Read the model definition and answer for the solid it produces. Units are mm, in the model's axes. A direction names the side the tool comes from. Coordinates: 2 decimals unless noted, no trailing zeros. Loops run counter-clockwise (first coordinate to the right, second up) from the corner with the lowest first, then second, coordinate; pieces in that order, holes last. Notation, with made-up numbers: (62, 62.5) - (120, 62.5) arc R13 cw to (120, 73.5) - close; hole circle Ø7 at (69.5, 77.5). An arc over 180 degrees is marked (long way). Use one line per item in the form item = value. Start each with the question number.
1) Each of these flat-tipped pins is pushed along its axis until it touches: P1, Ø1.5, axis at y = 1, z = 0, coming from the +X side; P2, Ø1.2, axis at x = 8.5, y = 2, coming from the -Z side. Where does it stop, or does it pass through?
2) The mould has two halves that part along X. Classify faces 1 (the face through (-2.017, 2.028, 9.283)), 2 (the face through (-0.397, 1.972, -17.024)), 3 (the face through (5.046, 1.972, -12.871)): released by +X, released by -X, zero draft, split by the parting line, or undercut.
3) Which of the six approach directions +Z, -Z, +X, -X, +Y, -Y give full straight-line access (tool end or side, diameter ignored) to faces 4 (the face through (9.56, 2.03, -6.91)), 5 (the face through (-5.11, 2.03, -0.39)), 6 (the face through (8, 2, -10.309))?
4) A cutting plane is placed at D-D (z = 5.75). Give the vertices of the cut face in (x, y), and give its area (3 significant figures).
5) A cutting plane is placed at C-C (x = -5.75). Give the vertices of the cut face in (y, z), and give its area (3 significant figures).
6) A cutting plane is placed at A-A (z = 0). Give the vertices of the cut face in (x, y).
7) A cutting plane is placed at B-B (y = 2.45). Give the vertices of the cut face in (x, z), and give its area (3 significant figures).
8) Consider line 1 (X direction, y = 0.9, z = 0); line 2 (Z direction, x = 0, y = 2.85); line 3 (Z direction, x = 0.5, y = 0.2). Determine where each line is inside the solid, lowest interval first.
from build123d import *

# Parameters (mm, degrees)
SKETCH1_R           = 3.05
SKETCH1_R_2         = 2.5
BOSS_EXTRUDE1_DEPTH = 4
SKETCH2_R           = 1.3
CUT_EXTRUDE1_DEPTH  = 4
SKETCH3_R           = 7.65
BOSS_EXTRUDE2_DEPTH = 4
BOSS_EXTRUDE3_DEPTH = 4
FILLET9_R           = 0.5


with BuildPart() as part:
    # Sketch1 → Boss-Extrude1 (new body)
    with BuildSketch(Plane(origin=(0, 0, 0), x_dir=(1, 0, 0), z_dir=(0, 1, 0))):
        with BuildLine():
            Line((-4.488689239, 15.114947499), (-7.764071496, 1.928521143))
            ThreePointArc((-7.764071496, 1.928521143), (0, -8), (7.764071496, 1.928521143))
            Line((7.764071496, 1.928521143), (4.488689239, 15.114947499))
            ThreePointArc((4.488689239, 15.114947499), (0, 18.625088), (-4.488689239, 15.114947499))
        make_face()
        with Locations((0, 14)):
            Circle(SKETCH1_R, mode=Mode.SUBTRACT)
        Circle(SKETCH1_R_2, mode=Mode.SUBTRACT)
    extrude(amount=BOSS_EXTRUDE1_DEPTH)

    # Sketch2 → Cut-Extrude1 (cut)
    with BuildSketch(Plane(origin=(0, 4, 0), x_dir=(1, 0, 0), z_dir=(0, 1, 0))):
        with Locations((0, 6.35)):
            Circle(SKETCH2_R)
        with Locations((6.35, 0)):
            Circle(SKETCH2_R)
        with Locations((0, -6.35)):
            Circle(SKETCH2_R)
        with Locations((-6.35, 0)):
            Circle(SKETCH2_R)
    extrude(amount=-CUT_EXTRUDE1_DEPTH, mode=Mode.SUBTRACT)

    # Sketch3 → Boss-Extrude2 (add)
    with BuildSketch(Plane(origin=(0, 4, 0), x_dir=(1, 0, 0), z_dir=(0, 1, 0))):
        with BuildLine():
            ThreePointArc((-1.549317863, 9.3728125), (0, -9.5), (1.549317863, 9.3728125))
            ThreePointArc((1.549317863, 9.3728125), (0, 9.120322757), (-1.549317863, 9.3728125))
        make_face()
        Circle(SKETCH3_R, mode=Mode.SUBTRACT)
    extrude(amount=-BOSS_EXTRUDE2_DEPTH)

    # Sketch4 → Boss-Extrude3 (add)
    with BuildSketch(Plane(origin=(0, 4, 0), x_dir=(1, 0, 0), z_dir=(0, 1, 0))):
        with BuildLine():
            Line((10.767160229, 10.309478294), (8.567165836, 4.1053221))
            Line((8.567165836, 4.1053221), (2.165063509, 1.25))
            ThreePointArc((2.165063509, 1.25), (1.994303817, 1.507565019), (1.793071605, 1.742094779))
            Line((1.793071605, 1.742094779), (5.682321854, 10.309478294))
            Line((5.682321854, 10.309478294), (10.767160229, 10.309478294))
        make_face()
    extrude(amount=-BOSS_EXTRUDE3_DEPTH)

    # Fillet9
    fillet9_edges = [part.edges().sort_by_distance(p)[0] for p in [
        (5.682321854, 2, -10.309478294),
        (10.767160229, 2, -10.309478294),
    ]]
    fillet(fillet9_edges, radius=FILLET9_R)


solid = part.part
Found:
q1.P1 = 9.5
q1.P2 = -10.31
q2.face_1 = split by the parting line
q2.face_2 = undercut
q2.face_3 = released by +X
q3.face_4 = +X, +Y, -Y
q3.face_5 = +Y, -Y
q3.face_6 = -Z, +X, +Y, -Y
q4.outline = (-7.56, 0) - (-1.15, 0) - (-1.15, 4) - (-7.56, 4) - close; (1.15, 0) - (7.56, 0) - (7.56, 4) - (1.15, 4) - close
q4.area = 51.3 mm^2
q5.outline = (0, -10.04) - (4, -10.04) - (4, -1.15) - (0, -1.15) - close; (0, 1.15) - (4, 1.15) - (4, 7.56) - (0, 7.56) - close
q5.area = 61.2 mm^2
q6.outline = (-9.5, 0) - (-7.65, 0) - (-7.65, 4) - (-9.5, 4) - close; (-5.05, 0) - (-2.5, 0) - (-2.5, 4) - (-5.05, 4) - close; (2.5, 0) - (5.05, 0) - (5.05, 4) - (2.5, 4) - close; (7.65, 0) - (9.5, 0) - (9.5, 4) - (7.65, 4) - close
q7.outline = (-6.53, -6.9) - (-4.49, -15.11) arc R4.63 ccw to (4.49, -15.11) - (5.59, -10.69) arc R0.5 cw to (6.07, -10.31) - (10.06, -10.31) arc R0.5 ccw to (10.53, -9.64) - (8.57, -4.11) arc R9.5 ccw (long way) to start; hole circle Ø2.6 at (-6.35, 0); hole circle Ø6.1 at (0, -14); hole circle Ø5 at (0, 0); hole circle Ø2.6 at (0, -6.35); hole circle Ø2.6 at (0, 6.35); hole circle Ø2.6 at (6.35, 0)
q7.area = 322 mm^2
q8.line_1 = -9.5 to -7.65, -5.05 to -2.5, 2.5 to 5.05, 7.65 to 9.5
q8.line_2 = -18.63 to -17.05, -10.95 to -7.65, -5.05 to -2.5, 2.5 to 5.05, 7.65 to 9.5
q8.line_3 = -18.6 to -17.01, -10.99 to -7.55, -5.15 to -2.45, 2.45 to 5.15, 7.55 to 9.49
